Model file for the job. Use its own axes, mm. Face numbers are marked on the shaded views. A direction names the side the tool comes from. Coordinates: 2 decimals unless noted, no trailing zeros. Loops run counter-clockwise (first coordinate to the right, second up) from the corner with the lowest first, then second, coordinate; pieces in that order, holes last. Notation, with made-up numbers: M 51.5,43.25 L 70.5,43.25 A12 cw 70.5,65.25 Z; hole C 13.5,70.25 d9. An arc over 180 degrees is marked long. Write item = value, one per line. Start each with the question number.
Autodesk Inventor part; units mm, degrees
ref_plane "YZ Plane" through (0, 0, 0) normal (1, 0, 0) x (0, 1, 0)
ref_plane "XZ Plane" through (0, 0, 0) normal (0, 1, 0) x (-1, 0, 0)
ref_plane "XY Plane" through (0, 0, 0) normal (0, 0, 1) x (1, 0, 0)
sketch "Sketch1" plane through (0, 0, 0) normal (0, 1, 0) x (-1, 0, 0)
  line L0 (12.573, 6.223) -> (-12.573, 6.223)
  line L1 (-12.573, 6.223) -> (-12.573, -6.223)
  line L2 (-12.573, -6.223) -> (12.573, -6.223)
  line L3 (12.573, -6.223) -> (12.573, 6.223)
  point P0 (0, 0)
  dimension "d0" = 12.446
  dimension "d1" = 25.146
  dimension "d2" = 6.223
  dimension "d3" = 12.573
extrude "Extrusion1" add sketch "Sketch1" along normal blind 6.35
sketch "Sketch2" plane through (12.573, 0, 6.223) normal (1, 0, 0) x (0, 0, -1)
  line L0 (-6.477, 0) -> (18.923, 0)
  line L1 (18.923, 0) -> (18.923, 1.5875)
  line L2 (18.923, 1.5875) -> (-6.477, 1.5875)
  line L3 (-6.477, 1.5875) -> (-6.477, 0)
  line L4 (0, 0) -> (12.446, 0)
  line L5 (0, 0) -> (12.446, 0)
  line L6 (12.446, 0) -> (12.446, 6.35)
  line L7 (0, 6.35) -> (12.446, 6.35)
  line L8 (0, 0) -> (0, 6.35)
  point P0 (6.223, 0)
  point P1 (6.223, 0)
  dimension "d6" = 25.4
  dimension "d7" = 12.7
  dimension "d8" = 1.5875
extrude "Extrusion2" add sketch "Sketch2" along normal blind 50.8 contours L3 L2 L8 L0 | L8 L2 L6 L0 | L6 L2 L1 L0
sketch "Sketch3" plane through (12.573, 1.5875, -6.223) normal (0, 1, 0) x (1, 0, 0)
  line L0 (0, 6.477) -> (0, 0)
  line L1 (0, -12.446) -> (0, 0)
  line L2 (0, -12.446) -> (0, -18.923)
  line L3 (0, -18.923) -> (50.8, -18.923)
  line L4 (50.8, 6.477) -> (50.8, -18.923)
  line L5 (0, 6.477) -> (50.8, 6.477)
  line L6 (50.8, -25.273) -> (50.8, 12.827)
  line L7 (50.8, 12.827) -> (76.2, -6.223)
  line L8 (76.2, -6.223) -> (50.8, -25.273)
  point P0 (-12.573, -6.223)
  point P1 (50.8, -18.923)
  dimension "d11" = 38.1
  dimension "d12" = 6.35
  dimension "d13" = 12.7
  dimension "d14" = 12.7
  dimension "d15" = 25.4
  dimension "d16" = 50.8
  dimension "d17" = 50.8
extrude "Extrusion3" add sketch "Sketch3" against normal blind 1.5875 contours L6 L7 L8 L4
sketch "Sketch4" plane through (12.573, 1.5875, -6.223) normal (0, 1, 0) x (1, 0, 0)
  line L0 (0, 6.477) -> (0, 0)
  line L1 (0, -12.446) -> (0, 0)
  line L2 (0, -12.446) -> (0, -18.923)
  line L3 (0, -18.923) -> (50.8, -18.923)
  line L4 (50.8, -18.923) -> (50.8, -25.273)
  line L5 (50.8, -25.273) -> (76.2, -6.223)
  line L6 (76.2, -6.223) -> (50.8, 12.827)
  line L7 (50.8, 12.827) -> (50.8, 6.477)
  line L8 (0, 6.477) -> (50.8, 6.477)
  line L9 (53.34, 3.937) -> (53.34, 7.747)
  line L10 (53.34, 7.747) -> (71.9667, -6.223)
  line L11 (71.9667, -6.223) -> (53.34, -20.193)
  line L12 (53.34, -20.193) -> (53.34, -16.383)
  line L13 (53.34, -16.383) -> (2.54, -16.383)
  line L14 (2.54, -16.383) -> (2.54, -12.446)
  line L15 (2.54, -12.446) -> (2.54, 0)
  line L16 (2.54, 0) -> (2.54, 3.937)
  line L17 (2.54, 3.937) -> (53.34, 3.937)
  point P0 (-12.573, -6.223)
  dimension "d20" = 2.54
extrude "Extrusion4" add sketch "Sketch4" along normal blind 9.525
sketch "Sketch6" plane through (15.113, 1.5875, -10.16) normal (0, 1, 0) x (1, 0, 0)
  line L0 (4.7625, -8.5725) -> (58.7375, -8.5725)
  line L1 (58.7375, -8.5725) -> (58.7375, -11.7475)
  line L2 (58.7375, -11.7475) -> (4.7625, -11.7475)
  line L3 (4.7625, -11.7475) -> (4.7625, -8.5725)
  line L4 (-27.686, -3.937) -> (-27.686, -16.383)
  point P0 (-15.113, -10.16)
  point P1 (-27.686, -10.16)
  dimension "d23" = 3.175
  dimension "d24" = 1.5875
extrude "Extrusion5" cut sketch "Sketch6" against normal blind 9.525
equation "\"d17\" = d16"
properties part number "Part_5_ledholder"
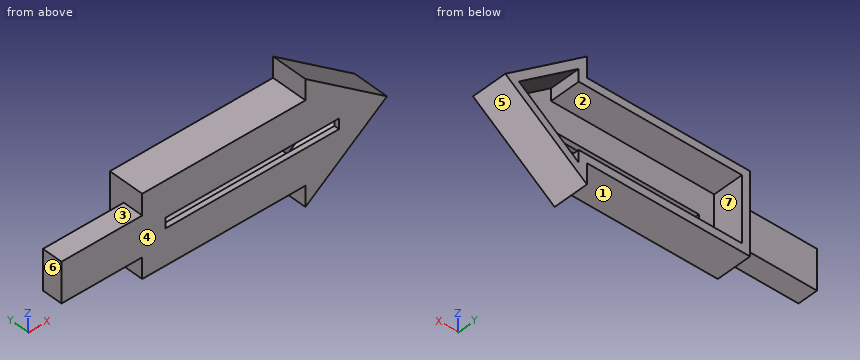
Item 1: Pull direction X, two halves, no side cores. Call the marked faces 4, 5, 6 and 7: +X half, -X half, draft (parallel to the pull), parting line (faces both ways), or undercut.
Item 2: Cut at C-C (z = -9). Give the cut face in (x, y).
Item 3: Probe L1, parallel to Z at x = 19, y = 2.75; L2, parallel to Y at x = 65.5, z = -10; L3, parallel to Z at x = 73.5, y = 4.25. List the from-to ranges inside material, lowest first.
Item 4: 3-axis set-ups, long thin cutter, end or side, ignore diameter. For the marked faces 1, 2 and 3: which of +Z, -Z, +X, -X, +Y, -Y reach the whole face in a straight line?
Item 5: Cut at A-A (x = 62). Give the cut face in (y, z), plus the area to 3 significant figures.
Item 6: Cut at B-B (y = 7.75). Give the cut face in (x, z), plus the area to 3 significant figures.
Item 7: Pin check, flat tips, straight feed: pin 1 Ø3 at (x, y) = (44, 5.5) entering from +Z; pin 2 Ø2 at (x, y) = (68, 9.5) entering from -Z; pin 3 Ø5 at (x, y) = (52, 6) entering from -Z. Stop position of each tip, or through.
Item 8: Cut at D-D (x = 81). Give the cut face in (y, z), plus the area to 3 significant figures.
Reported:
q1.face_4 = draft
q1.face_5 = +X half
q1.face_6 = -X half
q1.face_7 = undercut
q2.outline = M 12.57,0 L 76.77,0 L 76.77,11.11 L 72.54,11.11 L 72.54,1.59 L 15.11,1.59 L 15.11,11.11 L 12.57,11.11 Z
q3.L1 = -12.7 to -10.16, 10.16 to 12.7
q3.L2 = 0 to 1.59
q3.L3 = -11.45 to -8.28, 8.28 to 11.45
q4.face_1 = -Z, -X, +Y, -Y
q4.face_2 = +Y
q4.face_3 = +Z, -X, +Y, -Y
q5.outline = M 0,-12.7 L 11.11,-12.7 L 11.11,-10.16 L 1.59,-10.16 L 1.59,-1.59 L 0,-1.59 Z; M 0,1.59 L 1.59,1.59 L 1.59,10.16 L 11.11,10.16 L 11.11,12.7 L 0,12.7 Z
q5.area = 83.7 mm^2
q6.outline = M 12.57,-12.7 L 63.37,-12.7 L 63.37,-19.05 L 88.77,0 L 63.37,19.05 L 63.37,12.7 L 12.57,12.7 Z; hole M 15.11,-10.16 L 65.91,-10.16 L 65.91,-13.97 L 84.54,0 L 65.91,13.97 L 65.91,10.16 L 15.11,10.16 Z
q6.area = 482 mm^2
q7.pin_1 = 12.7
q7.pin_2 = -16.33
q7.pin_3 = -12.7
q8.outline = M 0,-5.83 L 11.11,-5.83 L 11.11,-2.65 L 1.59,-2.65 L 1.59,2.65 L 11.11,2.65 L 11.11,5.83 L 0,5.83 Z
q8.area = 79.0 mm^2
